```python
from build123d import *

# Parameters (mm, degrees)
F2_R    = 2.032
F3_SIZE = 0.762


with BuildPart() as f1:
    # F0 (on Front) → F1 (revolve)
    with BuildSketch(Plane.XZ):
        Polygon((-6.373, 65), (-6.373, 0), (-3.127, 0), (-3.127, 60), (0, 60), (0, 73), (-5, 73), align=None)
    revolve(axis=Axis((0, 0, 66.5), (0, 0, -1)))

    # F2
    f2_edges = [f1.edges().sort_by_distance(p)[0] for p in [
        (5, 0, 73),
    ]]
    fillet(f2_edges, radius=F2_R)

    # F3
    f3_edges = [f1.edges().sort_by_distance(p)[0] for p in [
        (3.127, 0, 0),
    ]]
    chamfer(f3_edges, length=F3_SIZE)


solid = f1.part
```
Part model, mm, in its own coordinate system. Round coordinates to 2 decimals unless told otherwise and drop trailing zeros. Order: outer loops, then holes, each group sorted by start corner. A loop starts at its lowest first (then second) coordinate and runs counter-clockwise, first axis right, second up. Notation, with made-up numbers: M 72,-30.5 L 78,-30.5 A24 ccw 78,-20.5 Z; hole C 71,-33.5 d10. An arc over 180 degrees is marked long. Put each result on its own line as item: value. Start each with the question number.
1. Drill centre lines: probe 1 along Y at (x, z) = (0.25, 29); probe 2 along Y at (x, z) = (0.25, 60.5); probe 3 along Y at (x, z) = (-2.75, 4). Where is each one in solid material? Low to high. Write a range as [from, to].
2. Drop flat-ended pins along their axis: pin 1 (3 mm diameter, centred on x = 0, y = 0.5, fed in from -Z); pin 2 (1 mm diameter, centred on x = -2, z = 43.5, fed in from +Y); pin 3 (2 mm diameter, centred on x = -1.5, z = 22.5, fed in from -Y). Give the stop position or say it passes through.
3. Slice it at A-A on y = 0. List the corners of the cut face in (x, z).
4. Slice it at C-C on z = 14. List the corners of the cut face in (x, y), then the cut area to 3 significant figures.
5. Two-plate mould, pull along Y, no slides. Class faces 1 (the face through (0.678, -3.053, 30.796)), 2 (the face through (1.38, -6.22, 32.04)), 3 (the face through (0, 0, 60)), 4 (the face through (3, -3, 0)): +Y half, -Y half, draft (parallel to the pull), parting line (faces both ways), or undercut.
Findings:
1. probe 1: [-6.37, -3.12], [3.12, 6.37]
1. probe 2: [-6.37, 6.37]
1. probe 3: [-5.75, -1.49], [1.49, 5.75]
2. pin 1: z = 60
2. pin 2: y = 6.19
2. pin 3: y = -6.35
3. outline: M -6.37,0 L -3.89,0 L -3.13,0.76 L -3.13,60 L 3.13,60 L 3.13,0.76 L 3.89,0 L 6.37,0 L 6.37,65 L 5.29,71.31 A2.03 ccw 3.29,73 L -3.29,73 A2.03 ccw -5.29,71.31 L -6.37,65 Z
4. outline: C 0,0 d12.75; hole C 0,0 d6.25
4. area: 96.9 mm2
5. face 1: undercut
5. face 2: parting line
5. face 3: undercut
5. face 4: draft
